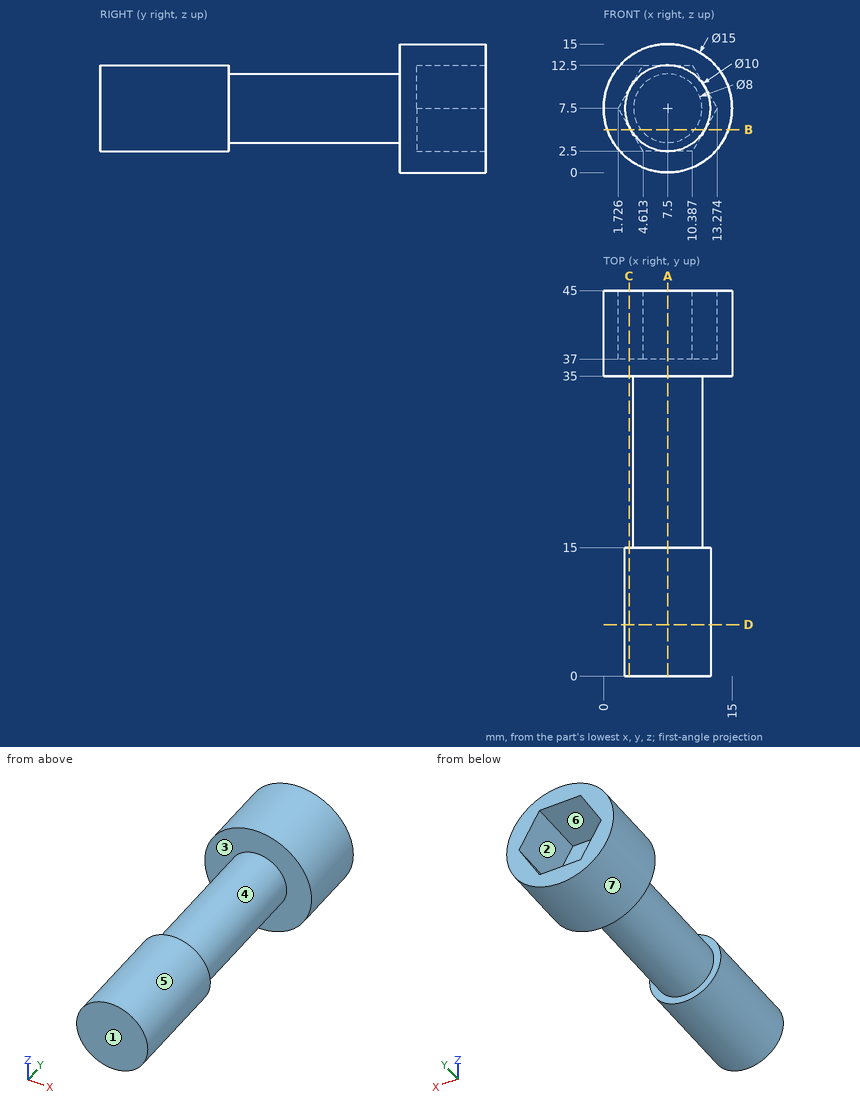
Geometry check sheet. Reference: drawing and pictorial views, mm from the part's lowest x, y, z. A direction names the side the tool comes from. Give positions to 0.01 mm unless a question says otherwise; leave off trailing zeros. Loops run counter-clockwise (first coordinate to the right, second up) from the corner with the lowest first, then second, coordinate; pieces in that order, holes last. Notation, with made-up numbers: (4, -13.5) -> (62, -13.5) arc R24 cw to (62, 1.5) -> close; hole circle Ø5 at (12, 32.5). An arc over 180 degrees is marked (long way). Answer in a Markdown table with one row per item. Add a question column.
1) Cross-section at D-D on y = 6. Record the boundary of the cut face in (x, z).
2) Set-up check for the marked faces 4, 5, 6 and 7: record each of +Z, -Z, +X, -X, +Y, -Y from which the full face is reachable in a straight line by a thin tool's end or side.
3) Cross-section at C-C on x = 3. Record the boundary of the cut face in (y, z) (1 decimal), and give its area (3 significant figures).
4) Cross-section at A-A on x = 7.5. Record the boundary of the cut face in (y, z), and give its area (3 significant figures).
5) Draft check along Y on the marked faces 1, 2 and 3. Enter one of: pulls with the +Y half, pulls with the -Y half, needs draft (parallel to the pull), parting line crosses it, or undercut.
6) Cross-section at B-B on z = 5. Record the boundary of the cut face in (x, y).
7) Material ranges on probe 1 along Y at (x, z) = (1.25, 6.25); probe 2 along X at (y, z) = (37.5, 5); probe 3 along Y at (x, z) = (8.25, 9.25), recorded low to high. Write a range as from..to.
8) Gauge pin test, flat ends, axial feed: P1, Ø1.5, axis at x = 4, y = 29.5, coming from the +Z side (1 decimal); P2, Ø3, axis at x = 9, y = 27.5, coming from the +Z side; P3, Ø6, axis at y = 17.5, z = 2.5, coming from the +X side. Record the tip position at first contact, or that the pin passes through.
Outcome:
| question | item | result |
|---|---|---|
| 1 | outline | circle Ø10 at (7.5, 7.5) |
| 2 | face 4 | none |
| 2 | face 5 | -Y |
| 2 | face 6 | +Y |
| 2 | face 7 | +Y, -Y |
| 3 | outline | (0, 5.3) -> (15, 5.3) -> (15, 9.7) -> (0, 9.7) -> close; (35, 1.5) -> (45, 1.5) -> (45, 5.3) -> (37, 5.3) -> (37, 9.7) -> (45, 9.7) -> (45, 13.5) -> (35, 13.5) -> close |
| 3 | area | 150 mm^2 |
| 4 | outline | (0, 2.5) -> (15, 2.5) -> (15, 3.5) -> (35, 3.5) -> (35, 0) -> (45, 0) -> (45, 2.5) -> (37, 2.5) -> (37, 12.5) -> (45, 12.5) -> (45, 15) -> (35, 15) -> (35, 11.5) -> (15, 11.5) -> (15, 12.5) -> (0, 12.5) -> close |
| 4 | area | 380 mm^2 |
| 5 | face 1 | pulls with the -Y half |
| 5 | face 2 | needs draft |
| 5 | face 3 | undercut |
| 6 | outline | (0.43, 35) -> (4.38, 35) -> (4.38, 15) -> (3.17, 15) -> (3.17, 0) -> (11.83, 0) -> (11.83, 15) -> (10.62, 15) -> (10.62, 35) -> (14.57, 35) -> (14.57, 45) -> (11.83, 45) -> (11.83, 37) -> (3.17, 37) -> (3.17, 45) -> (0.43, 45) -> close |
| 7 | probe 1 | y = 35..45 |
| 7 | probe 2 | x = 0.43..3.17, 11.83..14.57 |
| 7 | probe 3 | y = 0..37 |
| 8 | P1 | stops at z = 10.4 |
| 8 | P2 | stops at z = 11.5 |
| 8 | P3 | stops at x = 11.22 |
